The listing builds one solid part. Answer for the finished solid, in the listing's coordinates (mm). A direction names the side the tool comes from. Coordinates: 2 decimals unless noted, no trailing zeros. Loops run counter-clockwise (first coordinate to the right, second up) from the corner with the lowest first, then second, coordinate; pieces in that order, holes last. Notation, with made-up numbers: (3, 61) - (37, 61) arc R15 cw to (37, 79) - close; hole circle Ø9 at (86, -8). An arc over 180 degrees is marked (long way). Return JSON: item names as keys, results as strings. Group by question number.
1. Which of the six approach directions +Z, -Z, +X, -X, +Y, -Y give full straight-line access (tool end or side, diameter ignored) to faces 1 (the face through (649.3, -265.1, 77.3)), 2 (the face through (221, -233, 152.4)), 3 (the face through (-16, 88.9, 326))?
2. Each of these flat-tipped pins is pushed along its axis until it touches: P1, Ø5, axis at x = 426.5, z = 326, coming from the -Y side; P2, Ø1.5, axis at y = -232.5, z = 367, coming from the +X side; P3, Ø6, axis at y = -54.5, z = 209.5, coming from the -X side; P4, Ø12, axis at x = -604.5, y = 162.5, coming from the -Z side. Where does it stop, or does it pass through?
3. Section A-A (z = 692) is taken. Write down the section's boundary in (x, y), and give its area (3 significant figures).
4. The mould has two halves that part along Z. Classify faces 4 (the face through (-1142.908, 8.378, 375.666)), 5 (the face through (-204, 5, 0)), 6 (the face through (-544, 5, 762)): pulls with the +Z half, pulls with the -Z half, needs draft (parallel to the pull), parting line crosses it, or undercut.
5. Section B-B (y = 0) is taken. Write down the section's boundary in (x, z).
6. Section D-D (x = 206) is taken. Write down the section's boundary in (y, z), and give its area (3 significant figures).
7. Find the intervals of material crossed by line 1 along Y through (x, z) = (-762, 399); line 2 along Z through (x, y) = (142, -196); line 3 along Y through (x, z) = (-274.5, 340.5), in increasing order.
8. Section C-C (z = 63) is taken. Write down the section's boundary in (x, y), and give its area (3 significant figures).
```python
from build123d import *

# Parameters (mm, degrees)
F0_W     = 1524
F0_H     = 762
F1_DEPTH = 152.4
F2_W     = 457.2
F2_H     = 762
F3_DEPTH = 609.6
F5_DEPTH = 88.9
F6_R     = 190.5
F7_DEPTH = 1524
F9_DEPTH = 152.4


with BuildPart() as f1:
    # F0 (on Top) → F1 (new body)
    with BuildSketch(Plane.XY):
        Rectangle(F0_W, F0_H)
        with BuildLine():
            Line((-762, -381), (-762, 381))
            ThreePointArc((-762, 381), (-1143, 0), (-762, -381))
        make_face()
    extrude(amount=F1_DEPTH)

    # F2 (on face) → F3 (join)
    with BuildSketch(Plane.XY.offset(152.4)):
        with BuildLine():
            Line((-762, -381), (-762, 381))
            ThreePointArc((-762, 381), (-1143, 0), (-762, -381))
        make_face()
        with Locations((-533.4, 0)):
            Rectangle(F2_W, F2_H)
    extrude(amount=F3_DEPTH)

    # F4 (on Front) → F5 (join, symmetric)
    with BuildSketch(Plane.XZ):
        Polygon((762, 152.4), (-304.8, 762), (-304.8, 152.4), align=None)
    extrude(amount=F5_DEPTH, both=True)

    # F6 (on face) → F7 (cut)
    with BuildSketch(Plane.XY.offset(762)):
        with Locations((-762, 0)):
            Circle(F6_R)
    extrude(amount=-F7_DEPTH, mode=Mode.SUBTRACT)

    # F8 (on face) → F9 (cut)
    with BuildSketch(Plane.XY.offset(152.4)):
        Polygon((762, 381), (533.4, 381), (762, 152.4), align=None)
        Polygon((762, -381), (762, -152.4), (533.4, -381), align=None)
    extrude(amount=-F9_DEPTH, mode=Mode.SUBTRACT)


solid = f1.part
```
The answers:
{
 "1": {"face 1": "+Z, -Z, +X, -Y", "face 2": "+Z, +X, -Y", "face 3": "+Z, +X, +Y"},
 "2": {"P1": "stops at y = -88.9", "P2": "stops at x = -304.8", "P3": "stops at x = -1139.5", "P4": "stops at z = 0"},
 "3": {"outline": "(-762, -381) - (-304.8, -381) - (-304.8, -88.9) - (-182.3, -88.9) - (-182.3, 88.9) - (-304.8, 88.9) - (-304.8, 381) - (-762, 381) arc R381 ccw to start; hole circle Ø381 at (-762, 0)", "area": "484,000 mm2"},
 "4": {"face 4": "needs draft", "face 5": "pulls with the -Z half", "face 6": "pulls with the +Z half"},
 "5": {"outline": "(-1143, 0) - (-952.5, 0) - (-952.5, 762) - (-1143, 762) - close; (-571.5, 0) - (762, 0) - (762, 152.4) - (-304.8, 762) - (-571.5, 762) - close"},
 "6": {"outline": "(-381, 0) - (381, 0) - (381, 152.4) - (88.9, 152.4) - (88.9, 470.11) - (-88.9, 470.11) - (-88.9, 152.4) - (-381, 152.4) - close", "area": "173,000 mm2"},
 "7": {"line 1": "y = -381 to -190.5, 190.5 to 381", "line 2": "z = 0 to 152.4", "line 3": "y = -88.9 to 88.9"},
 "8": {"outline": "(-762, -381) - (533.4, -381) - (762, -152.4) - (762, 152.4) - (533.4, 381) - (-762, 381) arc R381 ccw to start; hole circle Ø381 at (-762, 0)", "area": "1,220,000 mm2"}
}
